CAD build for the part. Positions are in the model's coordinates, mm. Face numbers are marked on the shaded views. A direction names the side the tool comes from. Round coordinates to 2 decimals unless told otherwise and drop trailing zeros. Write each loop counter-clockwise with the first axis right and the second up, starting at its lowest first coordinate (ties: lowest second). Pieces come first, ordered by that corner, then holes. Notation, with made-up numbers: M 23,27 L 44,27 A28 cw 44,66 Z; hole C 53.5,40.5 d2. An arc over 180 degrees is marked long. Write each question's results on one line, items separated by ' | '. Start each with the question number.
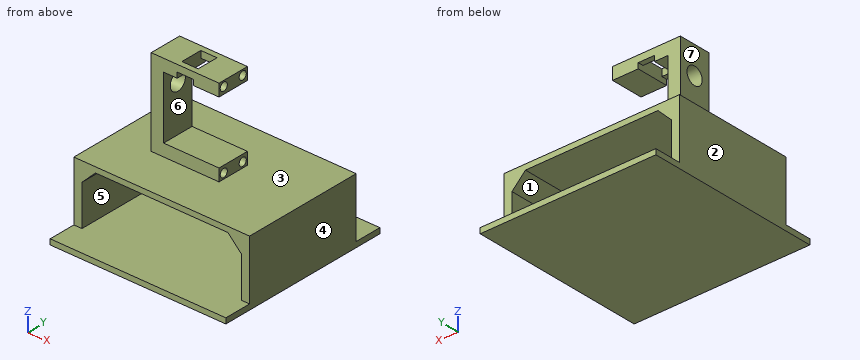
Autodesk Inventor part; units mm, degrees
ref_plane "YZ Plane" through (0, 0, 0) normal (1, 0, 0) x (0, 1, 0)
ref_plane "XZ Plane" through (0, 0, 0) normal (0, 1, 0) x (-1, 0, 0)
ref_plane "XY Plane" through (0, 0, 0) normal (0, 0, 1) x (1, 0, 0)
sketch "スケッチ1" plane through (0, 0, 0) normal (0, 0, 1) x (1, 0, 0)
  line L0 (-32.5, 32.5) -> (32.5, 32.5)
  line L1 (32.5, 32.5) -> (32.5, -32.5)
  line L2 (32.5, -32.5) -> (-32.5, -32.5)
  line L3 (-32.5, -32.5) -> (-32.5, 32.5)
  line L4 (-32.5, 32.5) -> (32.5, -32.5) construction
  line L5 (32.5, 32.5) -> (-32.5, -32.5) construction
  line L6 (-27, 27) -> (27, 27) construction
  line L7 (27, 27) -> (27, -27) construction
  line L8 (27, -27) -> (-27, -27) construction
  line L9 (-27, -27) -> (-27, 27) construction
  line L10 (-27, 27) -> (27, -27) construction
  line L11 (27, 27) -> (-27, -27) construction
  point P0 (0, 0)
  dimension "d0" = 65
  dimension "d1" = 65
  dimension "d2" = 54
  dimension "d3" = 54
extrude "押し出し1" add sketch "スケッチ1" along normal blind 2
sketch "スケッチ2" plane through (0, 0, 2) normal (0, 0, 1) x (1, 0, 0)
  line L0 (0, 54.4355) -> (0, -54.4355)
  line L1 (29.5, 22.5) -> (29.5, -22.5)
  line L2 (32.5, -32.5) -> (32.5, 32.5)
  line L3 (29.5, -22.5) -> (32.5, -22.5)
  line L4 (29.5, 22.5) -> (32.5, 22.5)
  line L5 (-36.7742, 0) -> (36.7742, 0)
  line L6 (-29.5, 22.5) -> (-29.5, -22.5)
  line L7 (-29.5, -22.5) -> (-32.5, -22.5)
  line L8 (-29.5, 22.5) -> (-32.5, 22.5)
  line L9 (-32.5, 32.5) -> (-32.5, -32.5)
  point P0 (0, 0)
  point P1 (32.5, 0)
  dimension "d7" = 22.5
  dimension "d8" = 45
  dimension "d9" = 3
extrude "押し出し2" add sketch "スケッチ2" along normal blind 20
sketch "スケッチ3" plane through (0, 0, 22) normal (0, 0, 1) x (1, 0, 0)
  line L0 (-32.5, -22.5) -> (-29.5, -22.5)
  line L1 (-29.5, -22.5) -> (-29.5, 22.5)
  line L2 (-29.5, 22.5) -> (-32.5, 22.5)
  line L3 (-32.5, 22.5) -> (-32.5, -22.5)
  line L4 (29.5, -22.5) -> (32.5, -22.5)
  line L5 (32.5, -22.5) -> (32.5, 22.5)
  line L6 (32.5, 22.5) -> (29.5, 22.5)
  line L7 (29.5, 22.5) -> (29.5, -22.5)
  line L8 (32.5, -22.5) -> (-32.5, -22.5)
  line L9 (-32.5, -22.5) -> (-32.5, 22.5)
  line L10 (-32.5, 22.5) -> (32.5, 22.5)
  line L11 (32.5, 22.5) -> (32.5, -22.5)
  point P0 (0, 0)
extrude "押し出し3" add sketch "スケッチ3" along normal blind 2
sketch "スケッチ4" plane through (0, 0, 24) normal (0, 0, 1) x (1, 0, 0)
  line L0 (13.75, -6) -> (-13.75, -6)
  line L1 (-13.75, -6) -> (-13.75, 6)
  line L2 (-13.75, 6) -> (13.75, 6)
  line L3 (13.75, 6) -> (13.75, -6)
  line L4 (13.75, -6) -> (-13.75, 6) construction
  line L5 (-13.75, -6) -> (13.75, 6) construction
  line L6 (-13.75, -6) -> (6.75, -6)
  line L7 (6.75, -6) -> (6.75, 6)
  line L8 (6.75, 6) -> (-13.75, 6)
  line L9 (-13.75, 6) -> (-13.75, -6)
  point P0 (0, 0)
  point P1 (6.75, -6)
  dimension "d14" = 27.5
  dimension "d15" = 12
  dimension "d16" = 7
extrude "押し出し4" add sketch "スケッチ4" along normal blind 4.5 contours L0 L1 L2 L7
sketch "スケッチ5" plane through (0, 0, 24) normal (0, 0, 1) x (1, 0, 0)
  line L0 (-13.75, -6) -> (-13.75, 6)
  line L1 (-13.75, -6) -> (-19.35, -6)
  line L2 (-19.35, -6) -> (-19.35, 6)
  line L3 (-19.35, 6) -> (-13.75, 6)
  line L4 (-13.75, 6) -> (-13.75, -6)
  line L5 (6.75, 6) -> (-13.75, 6)
  point P0 (0, 0)
  dimension "d19" = 5.6
extrude "押し出し5" add sketch "スケッチ5" along normal blind 32
sketch "スケッチ6" plane through (-13.75, -6, 28.5) normal (1, 0, 0) x (0, 0, -1)
  line L0 (0, 12) -> (0, 0)
  line L1 (0, 12) -> (-27.5, 12)
  line L2 (-27.5, 0) -> (-27.5, 12)
  line L3 (0, 0) -> (-27.5, 0)
  line L4 (-23, 0) -> (-23, 12)
  point P0 (28.5, 6)
  dimension "d22" = 4.5
extrude "押し出し6" add sketch "スケッチ6" along normal blind 20.5 contours L4 L3 L2 L1
sketch "スケッチ7" plane through (-19.35, -6, 24) normal (-1, 0, 0) x (0, 0, 1)
  line L0 (32, 12) -> (32, 0) construction
  line L1 (32, 6) -> (0, 6) construction
  line L2 (0, 28.5) -> (0, -16.5) construction
  point P0 (-24, 6)
  point P1 (21.79, 6)
  dimension "d25" = 10.21
hole "穴1" at (-19.35, 0, 45.79) direction (1, 0, 0) diameter 6.4 depth 6.3
sketch "スケッチ8" plane through (-19.35, -6, 24) normal (-1, 0, 0) x (0, 0, 1)
  circle A0 centre (21.79, 6) radius 3.2
  line L0 (0, 0) -> (0, 12)
  line L1 (0, 0) -> (32, 0)
  line L2 (32, 12) -> (32, 0)
  line L3 (0, 12) -> (32, 12)
  point P0 (-24, 6)
extrude "押し出し7" cut sketch "スケッチ8" against normal blind 1
sketch "スケッチ9" plane through (6.75, -6, 24) normal (1, 0, 0) x (0, 0, -1)
  circle A0 centre (-21.79, 6) radius 3.2
  line L0 (-58.0849, 6) -> (14.5049, 6)
  line L1 (0, -16.5) -> (0, 28.5)
  line L2 (-16, -14.4154) -> (-16, 26.4154)
  line L3 (-32, 12) -> (-32, 0)
  point P0 (24, 6)
  point P1 (-2, 2)
  point P2 (-2, 10)
  point P3 (-16, 6)
  point P4 (-30, 2)
  point P5 (-30, 10)
  dimension "d35" = 8
  dimension "d36" = 2
  dimension "d37" = 16
hole "穴2" at (6.75, -4, 26) at (6.75, 4, 26) at (6.75, -4, 54) at (6.75, 4, 54) direction (-1, 0, 0) diameter 3 depth 3
sketch "スケッチ10" plane through (0, 0, 2) normal (0, 0, 1) x (1, 0, 0)
  line L0 (24.25, -0.35) -> (-24.25, -0.35)
  line L1 (-24.25, -0.35) -> (-24.25, 28.35)
  line L2 (-24.25, 28.35) -> (24.25, 28.35)
  line L3 (24.25, 28.35) -> (24.25, -0.35)
  line L4 (24.25, -0.35) -> (-24.25, 28.35) construction
  line L5 (-24.25, -0.35) -> (24.25, 28.35) construction
  line L6 (32.5, 22.5) -> (32.5, 32.5)
  line L7 (32.5, 32.5) -> (-32.5, 32.5)
  circle A0 centre (24.25, -0.35) radius 3
  circle A1 centre (24.25, 28.35) radius 3
  circle A2 centre (-24.25, 28.35) radius 3
  circle A3 centre (-24.25, -0.35) radius 3
  point P0 (0, 0)
  point P1 (0, 14)
  point P2 (32.5, 27.5)
  dimension "d45" = 48.5
  dimension "d46" = 28.7
  dimension "d47" = 32.5
  dimension "d48" = 18.5
  dimension "d56" = 6
  dimension "d57" = 6
  dimension "d58" = 6
  dimension "d59" = 6
extrude "押し出し8" [suppressed]
sketch "スケッチ11" plane through (0, 0, 0) normal (0, 0, -1) x (-1, 0, 0)
  circle A0 centre (-24.25, 28.35) radius 3
  circle A1 centre (-24.25, -0.35) radius 3
  circle A2 centre (24.25, -0.35) radius 3
  circle A3 centre (24.25, 28.35) radius 3
  point P0 (0, 0)
  point P1 (-18.5, 30)
hole "穴4" [suppressed]
chamfer "面取り1" distance 5 angle 45 2 edges at (29.5, 0, 22) (-29.5, 0, 22)
fillet "フィレット1" [suppressed]
sketch "スケッチ12" plane through (0, 0, 56) normal (0, 0, 1) x (1, 0, 0)
  line L0 (-2.75, -4) -> (-8.75, -4)
  line L1 (-8.75, -4) -> (-8.75, 4)
  line L2 (-8.75, 4) -> (-2.75, 4)
  line L3 (-2.75, 4) -> (-2.75, -4)
  line L4 (-2.75, -4) -> (-8.75, 4) construction
  line L5 (-8.75, -4) -> (-2.75, 4) construction
  line L6 (-13.75, 6) -> (-13.75, -6)
  line L7 (-18.35, -6) -> (6.75, -6)
  point P0 (0, 0)
  point P1 (-5.75, 0)
  dimension "d73" = 6
  dimension "d74" = 8
  dimension "d75" = 5
  dimension "d76" = 6
extrude "押し出し9" cut sketch "スケッチ12" against normal blind 6.75
sketch "スケッチ13" plane through (6.75, 6, 28.5) normal (0, 1, 0) x (1, 0, 0)
  line L0 (-15.5, -23) -> (-9.5, -23)
  line L1 (-15.5, -23) -> (-9.5, -23)
  line L2 (-15.5, -27.5) -> (-15.5, -23)
  line L3 (-9.5, -27.5) -> (-15.5, -27.5)
  line L4 (-9.5, -27.5) -> (-9.5, -23)
  line L5 (-9.5, -25) -> (-15.5, -25)
  point P0 (-6.75, 28.5)
  dimension "d79" = 2
extrude "押し出し10" cut sketch "スケッチ13" against normal through all contours L0 L4 L5 L2
properties part number "Base"
1) 3-axis set-ups, long thin cutter, end or side, ignore diameter. For the marked faces 5, 6 and 7: which of +Z, -Z, +X, -X, +Y, -Y reach the whole face in a straight line?
2) Saw through at B-B, the plane y = 0. Write the cut outline in (x, z), plus the area to 3 significant figures.
3) Wall check: line 1 along Z through (x, y) = (6.1, 4); line 2 along Y through (x, z) = (4, 26); line 3 along Z through (x, y) = (18.5, -8). Give the ranges that are in metal, low to high. Write a range as from..to.
4) Saw through at A-A, the plane z = 10. Write the cut outline in (x, y), plus the area to 3 significant figures.
5) Saw through at D-D, the plane y = 7.5. Write the cut outline in (x, z), plus the area to 3 significant figures.
6) Saw through at C-C, the plane x = 15. Write the cut outline in (y, z), plus the area to 3 significant figures.
7) Drop flat-ended pins along their axis: pin 1 Ø2 at (x, y) = (19.5, 18) entering from -Z; pin 2 Ø0.8 at (x, z) = (-7, 54.5) entering from -Y; pin 3 Ø12 at (x, z) = (-6.5, 42.5) entering from +Y; pin 4 Ø1.5 at (y, z) = (4.5, 25.5) entering from +X. Give the stop position or say it passes through.
8) Pull direction X, two halves, no side cores. Call the marked faces 1, 2, 3 and 4: pulls with the +X half, pulls with the -X half, needs draft (parallel to the pull), parting line crosses it, or undercut.
Filled sheet:
1) face 5: +Y, -Y | face 6: +X, +Y, -Y | face 7: +Z, -X, +Y, -Y
2) outline: M -32.5,0 L 32.5,0 L 32.5,24 L 6.75,24 L 6.75,28.5 L -13.75,28.5 L -13.75,42.59 L -18.35,42.59 L -18.35,24 L -32.5,24 Z; M -18.35,48.99 L -13.75,48.99 L -13.75,51.5 L -8.75,51.5 L -8.75,56 L -18.35,56 Z; M -2.75,51.5 L 6.75,51.5 L 6.75,56 L -2.75,56 Z; hole M -29.5,2 L 29.5,2 L 29.5,17 L 24.5,22 L -24.5,22 L -29.5,17 Z | area: 680 mm^2
3) line 1: z = 0..2, 22..24.5, 27.5..28.5, 51.5..52.5, 55.5..56 | line 2: y = -6..-5.5, -2.5..2.5, 5.5..6 | line 3: z = 0..2, 22..24
4) outline: M -32.5,-22.5 L -29.5,-22.5 L -29.5,22.5 L -32.5,22.5 Z; M 29.5,-22.5 L 32.5,-22.5 L 32.5,22.5 L 29.5,22.5 Z | area: 270 mm^2
5) outline: M -32.5,0 L 32.5,0 L 32.5,24 L -32.5,24 Z; hole M -29.5,2 L 29.5,2 L 29.5,17 L 24.5,22 L -24.5,22 L -29.5,17 Z | area: 405 mm^2
6) outline: M -32.5,0 L 32.5,0 L 32.5,2 L -32.5,2 Z; M -22.5,22 L 22.5,22 L 22.5,24 L -22.5,24 Z | area: 220 mm^2
7) pin 1: stops at z = 0 | pin 2: stops at y = -6 | pin 3: passes through | pin 4: stops at x = 3.75
8) face 1: undercut | face 2: pulls with the -X half | face 3: needs draft | face 4: pulls with the +X half
